from build123d import *

# Parameters (mm, degrees)
SKETCH_1_R          = 2.05
EXTRUDE_1_DEPTH     = 5
SKETCH_2_R          = 4.05
CUT_EXTRUDE_1_DEPTH = 10
SKETCH_3_W          = 5
SKETCH_3_H          = 15
CUT_EXTRUDE_2_DEPTH = 153.47950682
EXTRUDE_2_DEPTH     = 5


with BuildPart() as part:
    # 草圖1 → 填料-伸長1 (new body)
    with BuildSketch(Plane(origin=(0, 0, 0), x_dir=(0, 0, -1), z_dir=(1, 0, 0))):
        Polygon((-70, -90), (-100, -90), (-100, 90), (100, 90), (100, -90), (70, -90), (70, -115), (50, -115), (50, -90), (10, -90), (10, -115), (-10, -115), (-10, -90), (-50, -90), (-50, -115), (-70, -115), align=None)
        with Locations((-60, -105)):
            Circle(SKETCH_1_R, mode=Mode.SUBTRACT)
        with Locations((0, -105)):
            Circle(SKETCH_1_R, mode=Mode.SUBTRACT)
        with Locations((60, -105)):
            Circle(SKETCH_1_R, mode=Mode.SUBTRACT)
    extrude(amount=EXTRUDE_1_DEPTH)

    # 草圖2 → 除料-伸長1 (cut)
    with BuildSketch(Plane(origin=(5, 0, 0), x_dir=(0, 0, -1), z_dir=(1, 0, 0))):
        with Locations((-10, 10)):
            Circle(SKETCH_2_R)
    extrude(amount=-CUT_EXTRUDE_1_DEPTH, mode=Mode.SUBTRACT)

    # 草圖3 → 除料-伸長2 (cut, through all)
    with BuildSketch(Plane(origin=(5, 0, 0), x_dir=(0, 0, -1), z_dir=(1, 0, 0))):
        with Locations((85.5, -47.5)):
            Rectangle(SKETCH_3_W, SKETCH_3_H)
        with Locations((85.5, -82.5)):
            Rectangle(SKETCH_3_W, SKETCH_3_H)
    extrude(amount=-CUT_EXTRUDE_2_DEPTH, mode=Mode.SUBTRACT)

    # 草圖4 → 填料-伸長2 (add)
    with BuildSketch(Plane.ZY):
        Polygon((-100, 90), (-350, 90), (-350, 60), (-130, -90), (-100, -90), align=None)
        Polygon((-130, 60), (-130, -53.69038103), (-296.745892177, 60), align=None, mode=Mode.SUBTRACT)
    extrude(amount=-EXTRUDE_2_DEPTH)


solid = part.part
CAD build for the part. Positions are in the model's coordinates, mm. A direction names the side the tool comes from. Round coordinates to 2 decimals unless told otherwise and drop trailing zeros. Loops run counter-clockwise (first coordinate to the right, second up) from the corner with the lowest first, then second, coordinate; pieces in that order, holes last.
(1) Which spindle directions (+Z, -Z, +X, -X, +Y, -Y) get a long thin tool onto all of the face, cutting with end or side? Do faces 4 (the flat face through (2.46, 2.36, -212.21)), 5 (the flat face through (0, 12, -78)). Say none if no direction does.
(2) Cut at B-B (y = -36). Give the cut face in (x, z), plus the area to 3 significant figures.
(3) Drop flat-ended pins along their axis: pin 1 (2.5 mm diameter, centred on x = 3, y = -101.5, fed in from +Z); pin 2 (2 mm diameter, centred on x = 0.5, y = -89, fed in from -Z); pin 3 (1.5 mm diameter, centred on x = 4.5, z = -188.5, fed in from -Y) (3 decimals). Give the stop position or say it passes through.
(4) Cut at D-D (y = -62). Give the cut face in (x, z).
(5) Wall check: line 1 along Z through (x, y) = (2.9, -98.5); line 2 along Y through (x, z) = (2.6, -60); line 3 along Z through (x, y) = (3.4, 59.5). Give the ranges that are in metal, low to high.
(6) Cut at C-C (z = -239). Give the cut face in (x, y), plus the area to 3 significant figures.
(7) Cut at A-A (x = 2.35). State how many separate pieces and enclosed holes the cut face has, plus the area to 3 significant figures.
(8) Two-plate mould, pull along Y, no slides. Class faces 1 (the flat face through (2.46, -13.95, -241.54)), 2 (the cylindrical face through (2.535, 7.536, 13.214)), 3 (the flat face through (5, 12, -78)): +Y half, -Y half, draft (parallel to the pull), parting line (faces both ways), or undercut.
Findings below:
1. face 4: +X, -X
1. face 5: +Z, -Z, -X, +Y, -Y
2. outline: (0, -209.2) - (5, -209.2) - (5, -155.95) - (0, -155.95) - close; (0, -130) - (5, -130) - (5, 100) - (0, 100) - close
2. area: 1,420 mm2
3. pin 1: stops at z = 70
3. pin 2: stops at z = -132.93
3. pin 3: stops at y = -50.625
4. outline: (0, -171.07) - (5, -171.07) - (5, 100) - (0, 100) - close
5. line 1: z = -70 to -50, -10 to 10, 50 to 70
5. line 2: y = -115 to -107.05, -102.95 to 90
5. line 3: z = -349.27 to -296.01, -130 to 100
6. outline: (0, -15.68) - (5, -15.68) - (5, 20.63) - (0, 20.63) - close; (0, 60) - (5, 60) - (5, 90) - (0, 90) - close
6. area: 332 mm2
7. separate pieces: 1
7. enclosed holes: 6
7. area: 56,300 mm2
8. face 1: -Y half
8. face 2: undercut
8. face 3: draft
